For this review, take the finished solid that the model builds, in its own axes (mm). Round coordinates to 2 decimals unless told otherwise and drop trailing zeros. Order: outer loops, then holes, each group sorted by start corner. A loop starts at its lowest first (then second) coordinate and runs counter-clockwise, first axis right, second up. Notation, with made-up numbers: M 8.5,84 L 35.5,84 A23 ccw 35.5,92 Z; hole C -29,5 d8. An arc over 180 degrees is marked long. Answer as a JSON object with one key per item and string values.
from build123d import *

# Parameters (mm, degrees)
SKETCH1_R           = 1.5
SKETCH1_R_2         = 3.5
BOSS_EXTRUDE1_DEPTH = 2


with BuildPart() as part:
    # Sketch1 → Boss-Extrude1 (new body)
    with BuildSketch(Plane.XY):
        with BuildLine():
            Line((-13, -14), (13, -14))
            Line((13, -14), (13, -7.331439149))
            ThreePointArc((13, -7.331439149), (10.5, 0), (13, 7.331439149))
            Line((13, 7.331439149), (13, 14))
            Line((13, 14), (-13, 14))
            Line((-13, 14), (-13, -14))
        make_face()
        with Locations((-8.357142857, 9)):
            Circle(SKETCH1_R, mode=Mode.SUBTRACT)
        with Locations((4, 0)):
            Circle(SKETCH1_R_2, mode=Mode.SUBTRACT)
        with Locations((3.642857143, 9)):
            Circle(SKETCH1_R, mode=Mode.SUBTRACT)
        with Locations((3.642857143, -9)):
            Circle(SKETCH1_R, mode=Mode.SUBTRACT)
        with Locations((-8.357142857, -9)):
            Circle(SKETCH1_R, mode=Mode.SUBTRACT)
    extrude(amount=BOSS_EXTRUDE1_DEPTH)


solid = part.part
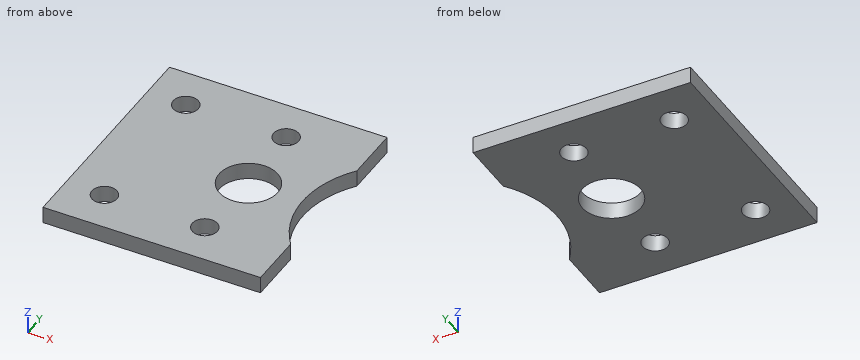
1) Add section A-A on y = 0. State the section outline as (x, z) points.
Geometry check:
{"outline": "M -13,0 L 0.5,0 L 0.5,2 L -13,2 Z; M 7.5,0 L 10.5,0 L 10.5,2 L 7.5,2 Z"}
2) Add section D-D on x = 4. State the section outline as (y, z) points.
Geometry check:
{"outline": "M -14,0 L -10.46,0 L -10.46,2 L -14,2 Z; M -7.54,0 L -3.5,0 L -3.5,2 L -7.54,2 Z; M 3.5,0 L 7.54,0 L 7.54,2 L 3.5,2 Z; M 10.46,0 L 14,0 L 14,2 L 10.46,2 Z"}
3) Add section B-B on z = 1.6. State the section outline as (x, y) points.
Geometry check:
{"outline": "M -13,-14 L 13,-14 L 13,-7.33 A12 cw 13,7.33 L 13,14 L -13,14 Z; hole C -8.36,-9 d3; hole C -8.36,9 d3; hole C 4,0 d7; hole C 3.64,-9 d3; hole C 3.64,9 d3"}
4) For L1, parallel to X at y = -10.25, z = 1.8; L2, parallel to X at y = 8, z = 0.55; L3, parallel to Y at x = 5, z = 1.3, list the stretches that pass through material, from the lowest coordinate up.
Geometry check:
{"L1": "x = -13 to -9.19, -7.53 to 2.81, 4.47 to 13", "L2": "x = -13 to -9.48, -7.24 to 2.52, 4.76 to 13", "L3": "y = -14 to -9.64, -8.36 to -3.35, 3.35 to 8.36, 9.64 to 14"}
5) Add section C-C on y = -9. State the section outline as (x, z) points.
Geometry check:
{"outline": "M -13,0 L -9.86,0 L -9.86,2 L -13,2 Z; M -6.86,0 L 2.14,0 L 2.14,2 L -6.86,2 Z; M 5.14,0 L 13,0 L 13,2 L 5.14,2 Z"}
